Part model, mm, in its own coordinate system. Give positions to 0.01 mm unless a question says otherwise; leave off trailing zeros. Write each loop counter-clockwise with the first axis right and the second up, starting at its lowest first coordinate (ties: lowest second). Pieces come first, ordered by that corner, then holes. Notation, with made-up numbers: (45, 26.25) - (85, 26.25) arc R26 ccw to (85, 65.25) - close; hole circle Ø2 at (-20.75, 44). An arc over 180 degrees is marked (long way). Answer as a JSON object with one key per item and string values. Group by question number.
```python
from build123d import *

# Parameters (mm, degrees)
BOSS_EXTRUDE1_DEPTH = 2


with BuildPart() as part:
    # Sketch1 → Boss-Extrude1 (new body)
    with BuildSketch(Plane(origin=(0, 0, 0), x_dir=(1, 0, 0), z_dir=(0, 1, 0))):
        Polygon((0, 0), (43, 0), (43, -2), (53, -2), (53, 0), (96, 0), (96, 18), (98, 18), (98, 23), (96, 23), (96, 41), (53, 41), (53, 43), (43, 43), (43, 41), (0, 41), align=None)
    extrude(amount=BOSS_EXTRUDE1_DEPTH)


solid = part.part
```
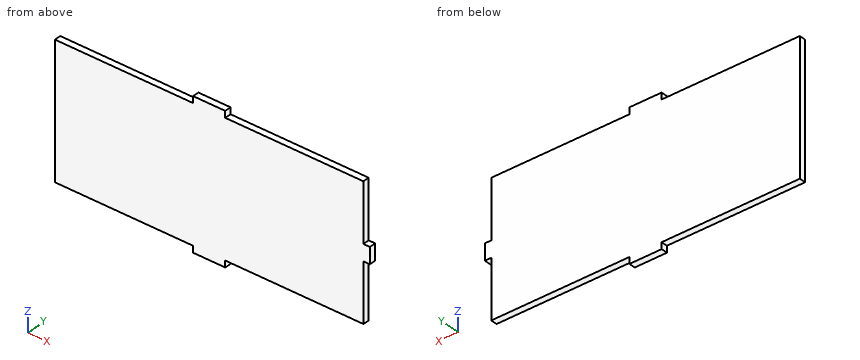
1) Drill centre lines: line 1 along Z through (x, y) = (71, 1.95); line 2 along X through (y, z) = (0.1, -10). Where is each one in solid material? Low to high. Write a range as from..to.
2) Saw through at B-B (x = 16). List the corners of the cut face in (y, z).
3) Drop flat-ended pins along their axis: P1, Ø8, axis at x = 80.5, z = -12, coming from the -Y side; P2, Ø0.6, axis at x = 65.5, y = 1, coming from the +Z side; P3, Ø0.6, axis at y = 1, z = 0.5, coming from the +X side; P4, Ø0.6, axis at x = 65.5, y = 1, coming from the -Z side. Give the stop position or say it passes through.
4) Saw through at A-A (y = 0.8). List the corners of the cut face in (x, z), and give its area (3 significant figures).
5) Saw through at C-C (z = -6.5). List the corners of the cut face in (x, y), and give its area (3 significant figures).
Checks:
{
 "1": {"line 1": "-41..0", "line 2": "0..96"},
 "2": {"outline": "(0, -41) - (2, -41) - (2, 0) - (0, 0) - close"},
 "3": {"P1": "y = 0", "P2": "z = 0", "P3": "x = 53", "P4": "z = -41"},
 "4": {"outline": "(0, -41) - (43, -41) - (43, -43) - (53, -43) - (53, -41) - (96, -41) - (96, -23) - (98, -23) - (98, -18) - (96, -18) - (96, 0) - (53, 0) - (53, 2) - (43, 2) - (43, 0) - (0, 0) - close", "area": "3,990 mm2"},
 "5": {"outline": "(0, 0) - (96, 0) - (96, 2) - (0, 2) - close", "area": "192 mm2"}
}
